Verification items for the finished model (mm, model axes). A direction names the side the tool comes from. Coordinates: 2 decimals unless noted, no trailing zeros. Order: outer loops, then holes, each group sorted by start corner. A loop starts at its lowest first (then second) coordinate and runs counter-clockwise, first axis right, second up. Notation, with made-up numbers: (46, 24) - (56, 24) arc R15 cw to (56, 52) - close; hole circle Ø6 at (-32.5, 70.25). An arc over 180 degrees is marked (long way). One line per question, with ' | ' between items. Start each with the question number.
from build123d import *

# Parameters (mm, degrees)
SKETCH_486_W        = 4.5
SKETCH_486_H        = 9
SKETCH_486_W_2      = 41
EXTRUDE_840_DEPTH   = 15
CUT_EXTRUDE_START   = 15
SKETCH_4_W          = 39
SKETCH_4_H          = 7
CUT_EXTRUDE_8_DEPTH = 10
SKETCH_5_W          = 4.5
SKETCH_5_H          = 6.901015062
CUT_EXTRUDE_9_DEPTH = 10


with BuildPart() as part:
    # Sketch 486 → Extrude 840 (new body)
    with BuildSketch(Plane(origin=(0, 0, 0), x_dir=(1, 0, 0), z_dir=(0, 1, 0))):
        Rectangle(SKETCH_486_W, SKETCH_486_H)
        Rectangle(SKETCH_486_W_2, SKETCH_486_H)
    extrude(amount=EXTRUDE_840_DEPTH)

    # 草图4 → 切除-拉伸8 (cut)
    with BuildSketch(Plane(origin=(0, 0, 0), x_dir=(1, 0, 0), z_dir=(0, 1, 0)).offset(CUT_EXTRUDE_START)):
        Rectangle(SKETCH_4_W, SKETCH_4_H)
    extrude(amount=-CUT_EXTRUDE_8_DEPTH, mode=Mode.SUBTRACT)

    # 草图5 → 切除-拉伸9 (cut)
    with BuildSketch(Plane(origin=(0, 15, 0), x_dir=(1, 0, 0), z_dir=(0, 1, 0))):
        with Locations((0, 3.450507531)):
            Rectangle(SKETCH_5_W, SKETCH_5_H)
    extrude(amount=-CUT_EXTRUDE_9_DEPTH, mode=Mode.SUBTRACT)


solid = part.part
Item 1: Mould release check, pull along Z, two halves, no side actions. Record for faces 4 (the flat face through (0, 10, 3.5)), 5 (the flat face through (0, 7, 4.5)), 6 (the flat face through (-2.25, 10, -4)): +Z half, -Z half, draft (parallel to the pull), parting line (faces both ways), or undercut.
Item 2: Section check C-C (z = -2.25). Record the cut outline in (x, y).
Item 3: Section check B-B (x = -12.5). Record the cut outline in (y, z).
Item 4: Section check A-A (y = 12.75). Record the cut outline in (x, z).
Item 5: Thickness scan on probe 1 along Z at (x, y) = (17.5, 11.75); probe 2 along X at (y, z) = (7.5, -2.5); probe 3 along Y at (x, z) = (-17.5, -3). Record the ranges inside material, lowest first. Write a range as from..to.
Item 6: Section check D-D (x = 0.5). Record the cut outline in (y, z), then the cut area to 3 significant figures.
Item 7: Set-up check for faces 1 (the flat face through (0, 4, -4.5)), 2 (the flat face through (11, 10, -3.5)), 3 (the flat face through (2.25, 10, -4)): record each of +Z, -Z, +X, -X, +Y, -Y from which the full face is reachable in a straight line by a thin tool's end or side.
Completed:
1) face 4: undercut | face 5: +Z half | face 6: draft
2) outline: (-20.5, 0) - (20.5, 0) - (20.5, 15) - (19.5, 15) - (19.5, 5) - (-19.5, 5) - (-19.5, 15) - (-20.5, 15) - close
3) outline: (0, -4.5) - (15, -4.5) - (15, -3.5) - (5, -3.5) - (5, 3.5) - (15, 3.5) - (15, 4.5) - (0, 4.5) - close
4) outline: (-20.5, -4.5) - (-2.25, -4.5) - (-2.25, -3.5) - (-19.5, -3.5) - (-19.5, 3.5) - (19.5, 3.5) - (19.5, -3.5) - (2.25, -3.5) - (2.25, -4.5) - (20.5, -4.5) - (20.5, 4.5) - (-20.5, 4.5) - close
5) probe 1: z = -4.5..-3.5, 3.5..4.5 | probe 2: x = -20.5..-19.5, 19.5..20.5 | probe 3: y = 0..5
6) outline: (0, -4.5) - (5, -4.5) - (5, 3.5) - (15, 3.5) - (15, 4.5) - (0, 4.5) - close | area: 55.0 mm^2
7) face 1: -Z, +X, -X, +Y, -Y | face 2: +Y | face 3: -Z, +Y
